```python
from build123d import *

# Parameters (mm, degrees)
F1_DEPTH  = 14
F3_D      = 9
F5_DEPTH  = 25
F6_R      = 5.1010545076
F7_DEPTH  = 2
F9_D      = 5
F10_R     = 1
F8_R      = 2.5
F11_DEPTH = 7


with BuildPart() as f1:
    # F0 (on Top) → F1 (new body)
    with BuildSketch(Plane.XY):
        Polygon((15, 0), (-15, 0), (-11.5, -20.7062792408), (11.5, -20.7062792408), align=None)
    extrude(amount=F1_DEPTH)

    # F3 (through all)
    with Locations(Plane(origin=(0, 0, 0), x_dir=(-1, 0, 0), z_dir=(0, 1, 0))):
        with Locations((0, 7)):
            Hole(F3_D / 2)

    # F4 (on face) → F5 (cut)
    with BuildSketch(Plane.XY.offset(14)):
        with BuildLine():
            ThreePointArc((5.8079340548, -20.7062792408), (7.7979945969, -17.8824961592), (8.5, -14.5))
            ThreePointArc((8.5, -14.5), (-3.3824961592, -6.7020054031), (-5.8079340548, -20.7062792408))
            Line((-5.8079340548, -20.7062792408), (5.8079340548, -20.7062792408))
        make_face()
    extrude(amount=-F5_DEPTH, mode=Mode.SUBTRACT)

    # F6 (on face) → F7 (join)
    with BuildSketch(Plane(origin=(0, 0, 0), x_dir=(-1, 0, 0), z_dir=(0, 1, 0))):
        with Locations((0, 7)):
            Circle(F6_R)
    extrude(amount=-F7_DEPTH)

    # F9 (through all)
    with Locations(Plane(origin=(0, 0, 0), x_dir=(-1, 0, 0), z_dir=(0, 1, 0))):
        with Locations((0, 7)):
            Hole(F9_D / 2)

    # F10
    f10_edges = [f1.edges().sort_by_distance(p)[0] for p in [
        (-5.807934, -20.706279, 7),
        (5.807934, -20.706279, 7),
    ]]
    fillet(f10_edges, radius=F10_R)

    # F8 (on face) → F11 (join)
    with BuildSketch(Plane(origin=(0, 0, 0), x_dir=(-1, 0, 0), z_dir=(0, 1, 0))):
        with Locations((-11.5, 7)):
            Circle(F8_R)
    extrude(amount=F11_DEPTH)


solid = f1.part
```
Geometry check sheet. Reference: the model listing, model coordinates, mm. A direction names the side the tool comes from. Coordinates: 2 decimals unless noted, no trailing zeros. Order: outer loops, then holes, each group sorted by start corner. A loop starts at its lowest first (then second) coordinate and runs counter-clockwise, first axis right, second up.
Item 1: Depth check by flat-ended pin: pin 1 (3 mm diameter, centred on y = -17.5, z = 11, fed in from -X); pin 2 (1 mm diameter, centred on y = -1, z = 9.5, fed in from -X); pin 3 (5.5 mm diameter, centred on x = 0, z = 7, fed in from -Y); pin 4 (4.5 mm diameter, centred on x = 0, z = 7, fed in from +Y). Enter the tip coordinate at first touch or a pass-through.
Item 2: Section check D-D (z = 1.5). Enter the section's corners in (x, y), plus the area to 3 significant figures.
Item 3: Section check B-B (z = 8). Enter the section's corners in (x, y), plus the area to 3 significant figures.
Item 4: Mould release check, pull along Y, two halves, no side actions. Record for faces 4 (the flat face through (13.226, -10.498, 6.902)), 5 (the cylindrical face through (-7.06, -20.17, 6.9)), 6 (the cylindrical face through (13, 3, 5)): released by +Y, released by -Y, zero draft, split by the parting line, or undercut.
Item 5: Section check C-C (x = 12). Enter the section's corners in (y, z), plus the area to 3 significant figures.
Item 6: Tool access check on faces 1 (the flat face through (-0.2, -5.6, 0)), 2 (the flat face through (-2, -2, 5)), 3 (the cylindrical face through (7.07, -20.19, 6.9)). Record the directions out of +Z, -Z, +X, -X, +Y, -Y that give a thin tool (end or side, any length) a straight path to the whole face; none if there is none.
Item 7: Scan lines: line 1 along Z through (x, y) = (0, -5.45); line 2 along Z through (x, y) = (0, -1.5); line 3 along Y through (x, z) = (9.75, 3.25). Record each from-to range of solid material in increasing order.
Item 8: Section check A-A (x = 0). Enter the section's corners in (y, z).
Check sheet entries:
1. pin 1: stops at x = -12.3
1. pin 2: stops at x = -14.92
1. pin 3: stops at y = -2
1. pin 4: passes through
2. outline: (-15, 0) - (-11.5, -20.71) - (-7.95, -20.71) arc R1 ccw to (-7.11, -19.16) arc R8.5 cw (long way) to (7.11, -19.16) arc R1 ccw to (7.95, -20.71) - (11.5, -20.71) - (15, 0) - close
2. area: 338 mm2
3. outline: (-15, 0) - (-11.5, -20.71) - (-7.95, -20.71) arc R1 ccw to (-7.11, -19.16) arc R8.5 cw to (-4.39, -7.22) - (-4.39, -2) - (-2.29, -2) - (-2.29, 0) - close; (2.29, -2) - (4.39, -2) - (4.39, -7.22) arc R8.5 cw to (7.11, -19.16) arc R1 ccw to (7.95, -20.71) - (11.5, -20.71) - (15, 0) - (13.79, 0) - (13.79, 7) - (9.21, 7) - (9.21, 0) - (2.29, 0) - close
3. area: 323 mm2
4. face 4: released by -Y
4. face 5: undercut
4. face 6: zero draft
5. outline: (-17.75, 0) - (0, 0) - (0, 4.55) - (7, 4.55) - (7, 9.45) - (0, 9.45) - (0, 14) - (-17.75, 14) - close
5. area: 283 mm2
6. face 1: -Z, +X, -X, +Y, -Y
6. face 2: -Y
6. face 3: +Z, -Z
7. line 1: z = 0 to 2.5, 11.5 to 14
7. line 2: z = 0 to 4.5, 9.5 to 14
7. line 3: y = -20.71 to 0
8. outline: (-6, 0) - (0, 0) - (0, 4.5) - (-2, 4.5) - (-2, 2.5) - (-6, 2.5) - close; (-6, 11.5) - (-2, 11.5) - (-2, 9.5) - (0, 9.5) - (0, 14) - (-6, 14) - close
